Autodesk Fusion 360 part; units mm, degrees
sketch "Sketch2" plane through (0, 0, 0) normal (0, 0, 1) x (1, 0, 0)
  circle A0 centre (8.5, 12) radius 3.5
  line L0 (-25, 24) -> (-25, 36)
  line L1 (0, 0) -> (0, 24)
  line L2 (-25, 24) -> (0, 24)
  line L3 (-25, 36) -> (17, 36)
  circle A1 centre (-19, 30) radius 2.5
  circle A2 centre (8.5, 12) radius 6
  line L4 (18.25, 10.75) -> (15.75, 10.75)
  line L5 (15.75, 10.75) -> (15.75, 13.25)
  line L6 (15.75, 13.25) -> (18.25, 13.25)
  line L7 (18.25, 13.25) -> (18.25, 10.75)
  line L8 (18.25, 10.75) -> (15.75, 13.25) construction
  line L9 (15.75, 10.75) -> (18.25, 13.25) construction
  line L10 (0, 0) -> (-25, 0)
  line L11 (-25, 0) -> (-25, -12)
  line L12 (-25, -12) -> (17, -12)
  line L13 (17, -12) -> (17, 36)
  line L14 (8.5, 12) -> (17, 12) construction
  circle A3 centre (-19, -6) radius 2.5
  point P0 (17, 12)
  dimension "d16" = 7
  dimension "d20" = 12
  dimension "d21" = 25
  dimension "d22" = 12
  dimension "d23" = 5
  dimension "d25" = 12
  dimension "d30" = 2.5
  dimension "d31" = 2.5
  dimension "d34" = 6
  dimension "d35" = 6
  dimension "d36" = 12
  dimension "d37" = 25
  dimension "d38" = 17
  dimension "d39" = 8.5
  dimension "d40" = 5
  dimension "d41" = 6
  dimension "d42" = 6
extrude "Extrude3" add sketch "Sketch2" along normal blind 4 contours L0 L1 L2 L3 L4 L5 L6 L10 L11 L12 L13 | L4 L5 L6 L13 | A2
extrude "Extrude4" cut sketch "Sketch2" along normal blind 2.1 contours A2
extrude "Extrude5" cut sketch "Sketch2" along normal blind 4 contours L4 L5 L6 L13
fillet "Fillet1" radius 6 4 edges at (-25, 24, 2) (-25, 0, 2) (-25, -12, 2) (-25, 36, 2)
CAD build for the part. Positions are in the model's coordinates, mm. A direction names the side the tool comes from. Round coordinates to 2 decimals unless told otherwise and drop trailing zeros. Write each loop counter-clockwise with the first axis right and the second up, starting at its lowest first coordinate (ties: lowest second). Pieces come first, ordered by that corner, then holes. Notation, with made-up numbers: M 89,79 L 97,79 A7 ccw 97,91 Z; hole C -4,57.5 d3. An arc over 180 degrees is marked long. Put each result on its own line as item: value. Start each with the question number.
1) Drill centre lines: probe 1 along Y at (x, z) = (-19, 2.85); probe 2 along Y at (x, z) = (8.5, 3.4); probe 3 along X at (y, z) = (2, 1.3). Where is each one in solid material? Low to high. Write a range as [from, to].
2) Pin check, flat tip, straight feed: pin 1 Ø2 at (y, z) = (10, 1) entering from -X. Stop position of the tip, or through.
3) Saw through at D-D, the plane y = 2. Write the cut outline in (x, z), and give its area (3 significant figures).
4) Pull direction X, two halves, no side cores. Call faces 5 (the flat face through (0.4, 12.3, 4)), 6 (the flat face through (15.75, 12, 2)), 7 (the cylindrical face through (-23.196, 34.289, 2.028)), 8 (the cylindrical face through (5.7, 14.1, 3)): pulls with the +X half, pulls with the -X half, needs draft (parallel to the pull), parting line crosses it, or undercut.
5) Saw through at C-C, the plane x = -17.5. Write the cut outline in (y, z).
6) Saw through at B-B, the plane y = 12. Write the cut outline in (x, z), and give its area (3 significant figures).
7) Saw through at A-A, the plane x = -2.5. Write the cut outline in (y, z).
8) 3-axis set-ups, long thin cutter, end or side, ignore diameter. For faces 1 (the cylindrical face through (-23.196, -1.711, 2.028)), 2 (the flat face through (-1, 36, 2)), 3 (the flat face through (16, 10.75, 2)), 4 (the cylindrical face through (4.08, 7.94, 1.04)): which of +Z, -Z, +X, -X, +Y, -Y reach the whole face in a straight line?
Resolved:
1. probe 1: [-12, -8.5], [-3.5, 0], [24, 27.5], [32.5, 36]
1. probe 2: [-12, 8.5], [15.5, 36]
1. probe 3: [0, 17]
2. pin 1: x = 0
3. outline: M 0,0 L 17,0 L 17,4 L 0,4 Z
3. area: 68.0 mm²
4. face 5: needs draft
4. face 6: pulls with the +X half
4. face 7: pulls with the -X half
4. face 8: undercut
5. outline: M -12,0 L -8,0 L -8,4 L -12,4 Z; M -4,0 L 0,0 L 0,4 L -4,4 Z; M 24,0 L 28,0 L 28,4 L 24,4 Z; M 32,0 L 36,0 L 36,4 L 32,4 Z
6. outline: M 0,0 L 2.5,0 L 2.5,2.1 L 5,2.1 L 5,4 L 0,4 Z; M 12,2.1 L 14.5,2.1 L 14.5,0 L 15.75,0 L 15.75,4 L 12,4 Z
6. area: 24.5 mm²
7. outline: M -12,0 L 0,0 L 0,4 L -12,4 Z; M 24,0 L 36,0 L 36,4 L 24,4 Z
8. face 1: +Z, -Z, -X
8. face 2: +Z, -Z, +X, -X, +Y
8. face 3: +Z, -Z, +X
8. face 4: -Z
